Can you work these out from the model? Positions are in its coordinate system, mm. A direction names the side the tool comes from. Round coordinates to 2 decimals unless told otherwise and drop trailing zeros. Order: outer loops, then holes, each group sorted by start corner. A loop starts at its lowest first (then second) coordinate and runs counter-clockwise, first axis right, second up. Notation, with made-up numbers: (78, 15) -> (93, 15) arc R30 cw to (93, 46) -> close; hole circle Ø5 at (2.25, 12). An arc over 180 degrees is marked (long way). One line per item, written item: value.
Autodesk Inventor part; units mm, degrees
ref_plane "YZ Plane" through (0, 0, 0) normal (1, 0, 0) x (0, 1, 0)
ref_plane "XZ Plane" through (0, 0, 0) normal (0, 1, 0) x (-1, 0, 0)
ref_plane "XY Plane" through (0, 0, 0) normal (0, 0, 1) x (1, 0, 0)
sketch "Sketch1" plane through (0, 0, 0) normal (0, 0, 1) x (1, 0, 0)
  line L0 (0, 0) -> (150, 0)
  line L1 (150, 0) -> (150, 150)
  line L2 (150, 150) -> (0, 150)
  line L3 (0, 150) -> (0, 0)
  circle A0 centre (110, 40) radius 16.5
  circle A1 centre (60, 40) radius 2
  line L4 (60, 40) -> (60, 90)
  circle A2 centre (60, 90) radius 5
  dimension "d0" = 150
  dimension "d1" = 150
  dimension "d2" = 33
  dimension "d3" = 4
  dimension "d4" = 50
  dimension "d5" = 10
extrude "Extrusion1" add sketch "Sketch1" along normal blind 8
sketch "Sketch2" plane through (0, 0, 0) normal (0, 0, -1) x (-1, 0, 0)
  circle A0 centre (-110, 40) radius 18.5
  point P0 (0, 0)
  dimension "d8" = 37
extrude "Extrusion2" cut sketch "Sketch2" against normal blind 7
properties part number "cote gauche"
Q1. I want a section at B-B on y = 40. List the corners of the cut face in (x, z) for me, plus the area to 3 significant figures.
Answers below:
outline: (0, 0) -> (58, 0) -> (58, 8) -> (0, 8) -> close; (62, 0) -> (91.5, 0) -> (91.5, 7) -> (93.5, 7) -> (93.5, 8) -> (62, 8) -> close; (126.5, 7) -> (128.5, 7) -> (128.5, 0) -> (150, 0) -> (150, 8) -> (126.5, 8) -> close
area: 876 mm^2
Q2. Will this pin go through, and if not, where does the flat tip stop? pin 1 Ø6 at (x, y) = (60, 90) entering from +Z (3 decimals).
Answers below:
pin 1: through
Q3. I want a section at D-D on x = 119.5. List the corners of the cut face in (y, z) for me.
Answers below:
outline: (0, 0) -> (24.13, 0) -> (24.13, 7) -> (26.51, 7) -> (26.51, 8) -> (0, 8) -> close; (53.49, 7) -> (55.87, 7) -> (55.87, 0) -> (150, 0) -> (150, 8) -> (53.49, 8) -> close
Q4. I want a section at A-A on x = 60. List the corners of the cut face in (y, z) for me.
Answers below:
outline: (0, 0) -> (38, 0) -> (38, 8) -> (0, 8) -> close; (42, 0) -> (85, 0) -> (85, 8) -> (42, 8) -> close; (95, 0) -> (150, 0) -> (150, 8) -> (95, 8) -> close
Q5. Please list where these lines run through material, in increasing order: line 1 along Y through (x, z) = (60, 5.5); line 2 along Y through (x, z) = (110, 1.75); line 3 along Y through (x, z) = (110, 7.75).
Answers below:
line 1: 0 to 38, 42 to 85, 95 to 150
line 2: 0 to 21.5, 58.5 to 150
line 3: 0 to 23.5, 56.5 to 150
Q6. On a 3-axis mill with a long thin cutter (end or side, diameter ignored), from which of +Z, -Z, +X, -X, +Y, -Y can I reach the whole of each face in a straight line? I mean faces 1 (the face through (92.911, 32.914, 3.451)), 2 (the face through (150, 74, 4)). Say none if no direction works.
Answers below:
face 1: -Z
face 2: +Z, -Z, +X, +Y, -Y
Q7. We'd pull the mould along Y, two halves only. Please class faces 3 (the face through (96.906, 50.04, 7.493)), 4 (the face through (76, 150, 4)), 5 (the face through (74, 76, 8)): released by +Y, released by -Y, zero draft, split by the parting line, or undercut.
Answers below:
face 3: undercut
face 4: released by +Y
face 5: zero draft
Q8. I want a section at C-C on z = 3.5. List the corners of the cut face in (x, y) for me, plus the area to 3 significant figures.
Answers below:
outline: (0, 0) -> (150, 0) -> (150, 150) -> (0, 150) -> close; hole circle Ø10 at (60, 90); hole circle Ø4 at (60, 40); hole circle Ø37 at (110, 40)
area: 21,300 mm^2
